CAD build for the part. Positions are in the model's coordinates, mm. Face numbers are marked on the shaded views. Give positions to 0.01 mm unless a question says otherwise; leave off trailing zeros. Write each loop counter-clockwise with the first axis right and the second up, starting at its lowest first coordinate (ties: lowest second). Pieces come first, ordered by that corner, then holes. Notation, with made-up numbers: (-25, 5) -> (15, 5) arc R23 cw to (15, 29) -> close; hole circle Ø4 at (13, 87). An arc over 180 degrees is marked (long way). Answer as a JSON object with one key per item and string values.
```python
from build123d import *


# Not quite as in the source:
# - a fillet or chamfer that OpenCascade refuses, or shapes differently, is made with other operations: its cross-section is extruded or revolved along the edge and cut away or added
# - a feature names something its author has since deleted; it is built from what else it names


with BuildPart() as f1:
    # F0 (on Front) → F1 (revolve)
    with BuildSketch(Plane.XZ):
        with BuildLine():
            Line((-11, 13), (-11, 0))
            Line((-11, 0), (-7.7, 0))
            Line((-7.7, 0), (-8.1, 7.9899937422))
            ThreePointArc((-8.1, 7.9899937422), (-5.7275649276, 13.7175586698), (0, 16.0899937422))
            Line((0, 16.0899937422), (0, 17.2))
            ThreePointArc((0, 17.2), (-2.4667280394, 17.6003207651), (-4.680255449, 18.7601915949))
            ThreePointArc((-4.680255449, 18.7601915949), (-7.0630577198, 15.0275401408), (-11, 13))
        make_face()
        with BuildLine():
            ThreePointArc((0, 32.8), (-7.3996792349, 27.4667280394), (-4.680255449, 18.7601915949))
            ThreePointArc((-4.680255449, 18.7601915949), (-2.4667280394, 17.6003207651), (0, 17.2))
            Line((0, 17.2), (0, 32.8))
        make_face()
    revolve(axis=Axis((0, 0, 29.5921396464), (0, 0, 1)))

    # F2: chamfer of 2 x 1 on 1 edges, made by hand

    # F2_s1 → F2_t2 (revolve, cut)
    with BuildSketch(Plane.XZ):
        Polygon((-8.7, 0), (-7.8, 1.9974984355), (-7.7, 0), align=None)
    revolve(axis=Axis((0, 0, 0), (0, 0, 1)), mode=Mode.SUBTRACT)


solid = f1.part
```
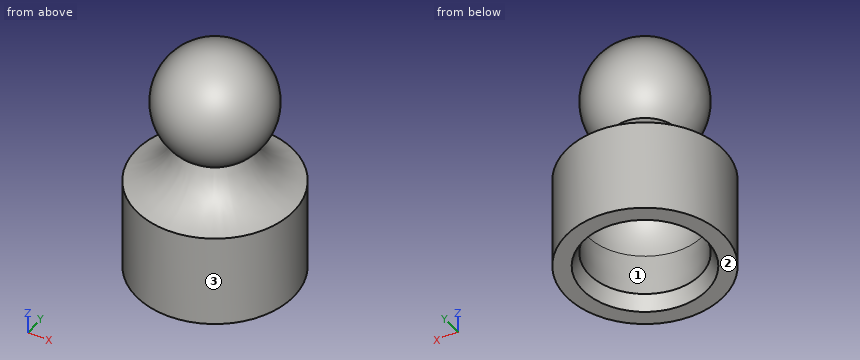
1) Wall check: probe 1 along Z at (x, y) = (1, 7); probe 2 along X at (y, z) = (1.5, 14); probe 3 along Z at (x, y) = (-2.75, -4.25). Give the ranges that are in metal, low to high.
Model answer:
{"probe 1": "z = 11.94 to 15.02, 21.71 to 28.29", "probe 2": "x = -8.32 to -5.22, 5.22 to 8.32", "probe 3": "z = 14.31 to 17.77, 19.07 to 30.93"}
2) Pin check, flat tips, straight feed: pin 1 (5 mm diameter, centred on x = -2.5, y = 1.5, fed in from +Z); pin 2 (2 mm diameter, centred on x = 3, z = 5.5, fed in from -Y); pin 3 (10 mm diameter, centred on y = 7.5, z = 17.5, fed in from +X). Stop position of each tip, or through.
Model answer:
{"pin 1": "stops at z = 32.79", "pin 2": "stops at y = -10.82", "pin 3": "stops at x = 9.63"}
3) Slice it at A-A (y = 0). List the corners of the cut face in (x, z), then the cut area to 3 significant figures.
Model answer:
{"outline": "(-11, 0) -> (-8.7, 0) -> (-7.8, 2) -> (-8.1, 7.99) arc R8.1 cw to (8.1, 7.99) -> (7.8, 2) -> (8.7, 0) -> (11, 0) -> (11, 13) arc R8.5 cw to (4.68, 18.76) arc R7.8 ccw (long way) to (-4.68, 18.76) arc R8.5 cw to (-11, 13) -> close", "area": "313 mm2"}
4) Slice it at D-D (z = 18). List the corners of the cut face in (x, y), then the cut area to 3 significant figures.
Model answer:
{"outline": "circle Ø9.92 at (0, 0)", "area": "77.3 mm2"}
5) Mould opens along X. For the marked faces 1, 2 and 3 say: released by +X, released by -X, zero draft, split by the parting line, or undercut.
Model answer:
{"face 1": "undercut", "face 2": "zero draft", "face 3": "split by the parting line"}
6) Slice it at C-C (z = 6.5). List the corners of the cut face in (x, y), then the cut area to 3 significant figures.
Model answer:
{"outline": "circle Ø22 at (0, 0); hole circle Ø16.05 at (0, 0)", "area": "178 mm2"}
